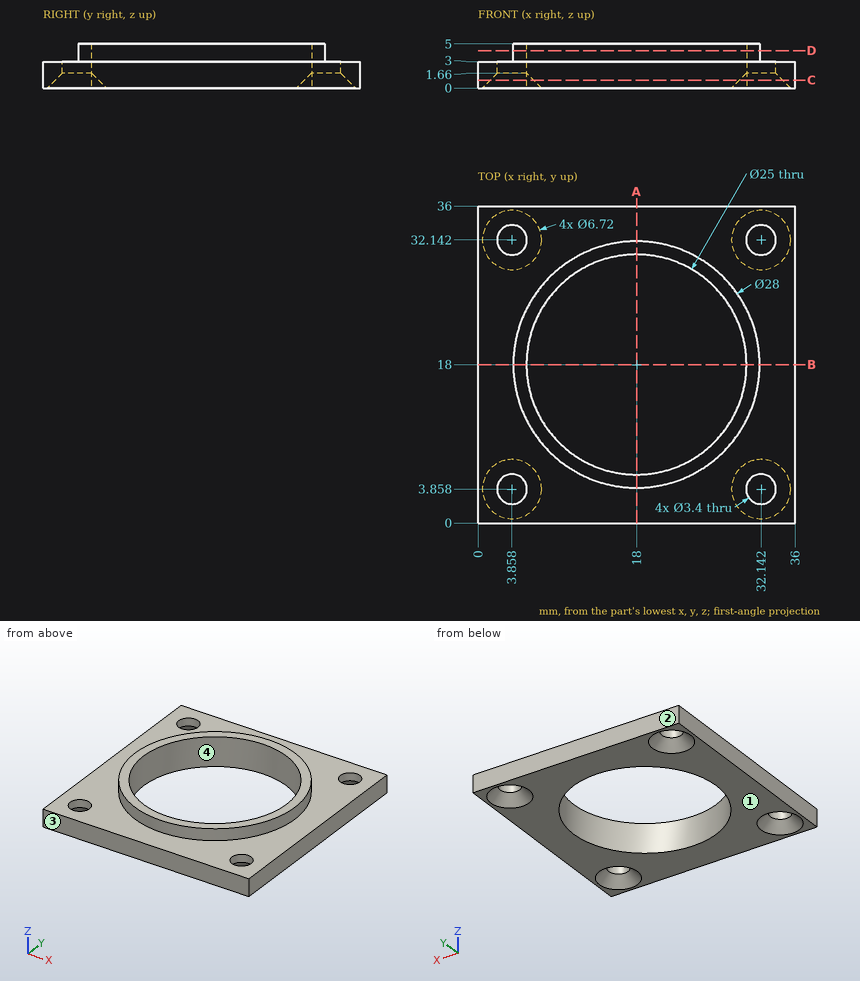
Source: three-view drawing plus pictorial views. Frame: mm from the lowest corner of the part. Round coordinates to 2 decimals unless told otherwise and drop trailing zeros. Order: outer loops, then holes, each group sorted by start corner. A loop starts at its lowest first (then second) coordinate and runs counter-clockwise, first axis right, second up. Notation, with made-up numbers: (-16.5, -32) - (33.5, -32) arc R22 cw to (33.5, 0) - close; hole circle Ø10 at (43, 45.25). An arc over 180 degrees is marked (long way). Answer in a Markdown table with one row per item.
Item 1: Section query C-C (z = 0.9). Return the cut outline in (x, y).
Model answer:
| item | result |
|---|---|
| outline | (0, 0) - (36, 0) - (36, 36) - (0, 36) - close; hole circle Ø4.92 at (3.86, 3.86); hole circle Ø4.92 at (3.86, 32.14); hole circle Ø25 at (18, 18); hole circle Ø4.92 at (32.14, 3.86); hole circle Ø4.92 at (32.14, 32.14) |
Item 2: Pin query (flat end, axial travel): pin 1 (4.5 mm diameter, centred on x = 32.14, y = 32.14, fed in from -Z); pin 2 (2 mm diameter, centred on x = 25.5, y = 12, fed in from -Z); pin 3 (4.5 mm diameter, centred on x = 3.86, y = 3.86, fed in from +Z). Return the tip coordinate at first contact, or that it passes through.
Model answer:
| item | result |
|---|---|
| pin 1 | stops at z = 1.11 |
| pin 2 | passes through |
| pin 3 | stops at z = 3 |
Item 3: Mould query, pull axis Y, two halves, no side actions, for the marked faces 1, 2, 3 and 4. Classes: released by +Y, released by -Y, zero draft, split by the parting line, or undercut.
Model answer:
| item | result |
|---|---|
| face 1 | zero draft |
| face 2 | released by +Y |
| face 3 | released by -Y |
| face 4 | undercut |
Item 4: Section query D-D (z = 4.25). Return the cut outline in (x, y).
Model answer:
| item | result |
|---|---|
| outline | circle Ø28 at (18, 18); hole circle Ø25 at (18, 18) |
Item 5: Section query A-A (x = 18). Return the cut outline in (y, z), then the cut area to 3 significant figures.
Model answer:
| item | result |
|---|---|
| outline | (0, 0) - (5.5, 0) - (5.5, 5) - (4, 5) - (4, 3) - (0, 3) - close; (30.5, 0) - (36, 0) - (36, 3) - (32, 3) - (32, 5) - (30.5, 5) - close |
| area | 39.0 mm² |
Item 6: Line query: line 1 (Y direction, x = 33, z = 2.9) (1 decimal); line 2 (Y direction, x = 18, z = 2); line 3 (Y direction, x = 33.5, z = 1.45) (1 decimal). Output: solid intervals per line, ascending.
Model answer:
| item | result |
|---|---|
| line 1 | y = 0 to 2.4, 5.3 to 30.7, 33.6 to 36 |
| line 2 | y = 0 to 5.5, 30.5 to 36 |
| line 3 | y = 0 to 2.5, 5.2 to 30.8, 33.5 to 36 |
